from build123d import *

# Parameters (mm, degrees)
ESQUISSE1_R             = 3.5
BOSS_EXTRU_1_DEPTH      = 50
ESQUISSE2_R             = 6.5
BOSS_EXTRU_2_DEPTH      = 2
CONG_1_R                = 1
ESQUISSE3_R             = 6
BOSS_EXTRU_3_DEPTH      = 20
ENL_V_START             = -11
ENL_V_MAT_EXTRU_1_DEPTH = 11
CONG_3_R                = 6
ESQUISSE5_R             = 2.5
ENL_V_MAT_EXTRU_2_DEPTH = 6


with BuildPart() as part:
    # Esquisse1 → Boss.-Extru.1 (new body)
    with BuildSketch(Plane.XY):
        Circle(ESQUISSE1_R)
    extrude(amount=BOSS_EXTRU_1_DEPTH)

    # Esquisse2 → Boss.-Extru.2 (add)
    with BuildSketch(Plane(origin=(0, 0, 0), x_dir=(-1, 0, 0), z_dir=(0, 0, -1))):
        Circle(ESQUISSE2_R)
    extrude(amount=BOSS_EXTRU_2_DEPTH)

    # Congé1
    cong_1_edges = [part.edges().sort_by_distance(p)[0] for p in [
        (6.5, 0, -2),
    ]]
    fillet(cong_1_edges, radius=CONG_1_R)

    # Esquisse3 → Boss.-Extru.3 (add)
    with BuildSketch(Plane(origin=(0, 0, -2), x_dir=(-1, 0, 0), z_dir=(0, 0, -1))):
        Circle(ESQUISSE3_R)
    extrude(amount=BOSS_EXTRU_3_DEPTH)

    # Esquisse4 → Enlèv. mat.-Extru.1 (cut)
    with BuildSketch(Plane(origin=(0, 0, -22), x_dir=(-1, 0, 0), z_dir=(0, 0, -1)).offset(ENL_V_START)):
        with BuildLine():
            Line((5.196152423, -3), (-5.196152423, -3))
            ThreePointArc((-5.196152423, -3), (0, -6), (5.196152423, -3))
        make_face()
        with BuildLine():
            ThreePointArc((5.196152423, 3), (0, 6), (-5.196152423, 3))
            Line((-5.196152423, 3), (5.196152423, 3))
        make_face()
    extrude(amount=ENL_V_MAT_EXTRU_1_DEPTH, mode=Mode.SUBTRACT)

    # Congé3
    # the kernel refuses this fillet: 6 mm, written as the material it takes off along each edge
    with BuildSketch(Plane(origin=(0, 0, -22), x_dir=(-0.9930943434085017, 0.11731847718938858, 0), z_dir=(-0.11731847718938858, -0.9930943434085017, 0))) as cong_3_piece_1:
        with BuildLine():
            CenterArc((0.0001, -5.9999), CONG_3_R, 0, 90)
            Line((0.0001, 0.0001), (0.0001, 0.1201))
            ThreePointArc((0.0001, 0.1201), (3.00005, 0.12), (6, 0.12))
            Line((6, 0.12), (6.12, 0))
            ThreePointArc((6.12, 0), (6.12, -2.99995), (6.1201, -5.9999))
            Line((6.1201, -5.9999), (6.0001, -5.9999))
        make_face()
    revolve(axis=Axis((0, 0, -22), (0, 0, -1)), revolution_arc=346.525261187, mode=Mode.SUBTRACT)
    with BuildSketch(Plane(origin=(0, 0, -22), x_dir=(-1, 0, 0), z_dir=(0, -1, 0))) as cong_3_piece_2:
        with BuildLine():
            CenterArc((0.0001, -5.9999), CONG_3_R, 0, 90)
            Line((0.0001, 0.0001), (0.0001, 0.1201))
            ThreePointArc((0.0001, 0.1201), (3.00005, 0.12), (6, 0.12))
            Line((6, 0.12), (6.12, 0))
            ThreePointArc((6.12, 0), (6.12, -2.99995), (6.1201, -5.9999))
            Line((6.1201, -5.9999), (6.0001, -5.9999))
        make_face()
    revolve(axis=Axis((0, 0, -22), (0, 0, -1)), revolution_arc=173.243453158, mode=Mode.SUBTRACT)
    with BuildSketch(Plane(origin=(0, 0, -22), x_dir=(0.9930550201853389, -0.11765086861003726, 0), z_dir=(0.11765086861003726, 0.9930550201853389, 0))) as cong_3_piece_3:
        with BuildLine():
            CenterArc((0.0001, -5.9999), CONG_3_R, 0, 90)
            Line((0.0001, 0.0001), (0.0001, 0.1201))
            ThreePointArc((0.0001, 0.1201), (3.00005, 0.12), (6, 0.12))
            Line((6, 0.12), (6.12, 0))
            ThreePointArc((6.12, 0), (6.12, -2.99995), (6.1201, -5.9999))
            Line((6.1201, -5.9999), (6.0001, -5.9999))
        make_face()
    revolve(axis=Axis((0, 0, -22), (0, 0, -1)), revolution_arc=173.243453158, mode=Mode.SUBTRACT)

    # Esquisse5 → Enlèv. mat.-Extru.2 (cut)
    with BuildSketch(Plane(origin=(0, 3, 0), x_dir=(1, 0, 0), z_dir=(0, 1, 0))):
        with Locations(Location((0, 16.359037674, 0), (0, 0, 180))):
            Circle(ESQUISSE5_R)
    extrude(amount=-ENL_V_MAT_EXTRU_2_DEPTH, mode=Mode.SUBTRACT)


solid = part.part
Could you check a few things on this model? Use its own coordinates, in mm. A direction names the side the tool comes from. Coordinates: 2 decimals unless noted, no trailing zeros. Write each loop counter-clockwise with the first axis right and the second up, starting at its lowest first coordinate (ties: lowest second). Pieces come first, ordered by that corner, then holes. Notation, with made-up numbers: (-10.75, 38) - (-4.75, 38) arc R19 ccw to (-4.75, 64) - close; hole circle Ø8 at (83, -15.5). An arc over 180 degrees is marked (long way). Put each result on its own line as item: value. Start each with the question number.
Q1. Thinking about a two-plate mould opening in Z: for faces 5 (the flat face through (1.1, -3, -13.8)), 6 (the cylindrical face through (0.33, 0.04, -13.88)), 7 (the flat face through (-3, -3, 0)), 8 (the flat face through (0, 4, -11)), which applies, pulls with the +Z half, pulls with the -Z half, needs draft (parallel to the pull), parting line crosses it, or undercut?
Q2. I want a section at A-A on z = 32. Write out the boundary of the cut face in (x, y).
Q3. I'm going to push flat-ended pins straight in: P1, Ø2.5, axis at x = -1.5, y = -4.5, coming from the -Z side; P2, Ø5, axis at x = -0.5, z = -15.5, coming from the +Y side; P3, Ø2, axis at x = 5, y = 4.5, coming from the +Z side; P4, Ø4.5, axis at x = 0, z = -16.36, coming from the +Y side. Where does each tip first touch, or does it pass through?
Q4. Which directions (+Z, -Z, +X, -X, +Y, -Y) give clear straight access to the entire face, cutting with the end or side of a thin tool? Please do faces 1 (the cylindrical face through (-5.54, -2.3, -7.36)), 2 (the flat face through (0, -4, -11)), 3 (the flat face through (-1.1, 3, -13.8)), 4 (the cylindrical face through (3.233, -1.341, 24.65)).
Q5. Please list where these lines run through material, in increasing order: L1, parallel to Z at x = 0, y = 1.2; L2, parallel to Z at x = 0, y = -0.65; L3, parallel to Z at x = -3, y = 4.5.
Checks:
1. face 5: needs draft
1. face 6: undercut
1. face 7: pulls with the +Z half
1. face 8: pulls with the -Z half
2. outline: circle Ø7 at (0, 0)
3. P1: z = -11
3. P2: y = 3
3. P3: z = 0
3. P4: through
4. face 1: -Z
4. face 2: -Z, +X, -X, -Y
4. face 3: -Z, +X, -X, +Y
4. face 4: +Z
5. L1: -21.88 to -18.86, -13.86 to 50
5. L2: -21.96 to -18.86, -13.86 to 50
5. L3: -11 to 0
